Source: CAD feature listing. Evaluate the final solid. Frame: model axes, mm. Face numbers are marked on the shaded views. A direction names the side the tool comes from. Coordinates: 2 decimals unless noted, no trailing zeros. Write item = value, one per line. Start each with the question number.
1. Access query for the marked faces 1, 2 and 3. Directions: +Z, -Z, +X, -X, +Y, -Y. A direction counts if a zero-diameter tool reaches every point of the face in a straight line with its end or side. Return the directions, or none.
2. Line query: line 1 along Y through (x, z) = (-13.8, -17.5) (3 decimals); line 2 along X through (y, z) = (-13, -18.75); line 3 along Y through (x, z) = (15, -20.5) (3 decimals). Output: solid intervals per line, ascending.
3. Pin query (flat end, axial travel): pin 1 Ø1.3 at (y, z) = (4.5, -17.5) entering from -X; pin 2 Ø10 at (x, y) = (8.5, -12) entering from +Z; pin 3 Ø2.5 at (x, y) = (-7.78, -7.78) entering from +Z; pin 4 Ø1.1 at (x, z) = (13, -18) entering from +Y. Return the tip coordinate at first contact, or that it passes through.
4. Section query A-A (y = -3.5). Give the number of separate pieces and of enclosed holes in the cut face, then the cut area to 3 significant figures.
```python
from build123d import *

# Parameters (mm, degrees)
BOSS_EXTRUDE1_DEPTH              = 4.5
BOSS_EXTRUDE2_DEPTH              = 1.5
SKETCH3_W                        = 34.4
SKETCH3_H                        = 6
BOSS_EXTRUDE3_DEPTH              = 16.965402213
SKETCH4_W                        = 4.5
SKETCH4_H                        = 18
CUT_EXTRUDE1_DEPTH               = 24.8
SKETCH5_W                        = 4.8
SKETCH5_H                        = 6
BOSS_EXTRUDE4_DEPTH              = 4
SKETCH6_W                        = 4.8
SKETCH6_H                        = 6
BOSS_EXTRUDE5_DEPTH              = 4
SKETCH7_W                        = 4.5
SKETCH7_H                        = 12
CUT_EXTRUDE2_DEPTH               = 3.6
SKETCH8_W                        = 3.6
SKETCH8_H                        = 12
CUT_EXTRUDE3_DEPTH               = 4.5
F_2_05_2_05_DIAMETER_HOLE1_D     = 2.05
F_2_05_2_05_DIAMETER_HOLE1_DEPTH = 4.8
F_2_05_2_05_DIAMETER_HOLE2_D     = 2.05
F_2_5_2_5_DIAMETER_HOLE1_D       = 2.5
F_2_05_2_05_DIAMETER_HOLE3_D     = 2.05
F_2_05_2_05_DIAMETER_HOLE3_DEPTH = 6.000025
F_1_6_1_6_DIAMETER_HOLE1_D       = 1.6
F_1_6_1_6_DIAMETER_HOLE1_DEPTH   = 6.000025
F_8_0_8_DIAMETER_HOLE1_D         = 8
F_2_05_2_05_DIAMETER_HOLE4_D     = 2.05
F_2_05_2_05_DIAMETER_HOLE4_DEPTH = 9.5
CHAMFER1_SIZE                    = 0.3
CHAMFER2_SIZE2                   = 0.199958733
CHAMFER2_SIZE                    = 0.19995667
CHAMFER3_SIZE                    = 0.18964074
CHAMFER3_SIZE_2                  = 0.224716875
FILLET1_R                        = 1.5
FILLET2_R                        = 2


with BuildPart() as part:
    # Sketch1 → Boss-Extrude1 (new body)
    with BuildSketch(Plane.XY.offset(-15)):
        with BuildLine():
            Line((-17.2, 5.965402213), (17.2, 5.965402213))
            Line((17.2, 5.965402213), (15.505698966, 7.387089586))
            ThreePointArc((15.505698966, 7.387089586), (15.038810903, 7.100113286), (14.5, 7))
            Line((14.5, 7), (-14.5, 7))
            ThreePointArc((-14.5, 7), (-15.038810903, 7.100113286), (-15.505698966, 7.387089586))
            Line((-15.505698966, 7.387089586), (-17.2, 5.965402213))
        make_face()
    extrude(amount=-BOSS_EXTRUDE1_DEPTH)

    # Sketch2 → Boss-Extrude2 (add)
    with BuildSketch(Plane(origin=(0, 0, -19.5), x_dir=(-1, 0, 0), z_dir=(0, 0, -1))):
        Polygon((17.2, 5.965402213), (-17.2, 5.965402213), (-11.2, 11), (11.2, 11), align=None)
    extrude(amount=BOSS_EXTRUDE2_DEPTH)

    # Sketch3 → Boss-Extrude3 (add)
    with BuildSketch(Plane.XZ.offset(-5.965402213)):
        with Locations((0, -18)):
            Rectangle(SKETCH3_W, SKETCH3_H)
    extrude(amount=BOSS_EXTRUDE3_DEPTH)

    # Sketch4 → Cut-Extrude1 (cut)
    with BuildSketch(Plane(origin=(12.4, 0, 0), x_dir=(0, 0, -1), z_dir=(1, 0, 0))):
        with Locations((17.25, -2)):
            Rectangle(SKETCH4_W, SKETCH4_H)
    extrude(amount=-CUT_EXTRUDE1_DEPTH, mode=Mode.SUBTRACT)

    # Sketch5 → Boss-Extrude4 (add)
    with BuildSketch(Plane.XZ.offset(11)):
        with Locations((14.8, -18)):
            Rectangle(SKETCH5_W, SKETCH5_H)
    extrude(amount=BOSS_EXTRUDE4_DEPTH)

    # Sketch6 → Boss-Extrude5 (add)
    with BuildSketch(Plane.XZ.offset(11)):
        with Locations((-14.8, -18)):
            Rectangle(SKETCH6_W, SKETCH6_H)
    extrude(amount=BOSS_EXTRUDE5_DEPTH)

    # Sketch7 → Cut-Extrude2 (cut)
    with BuildSketch(Plane(origin=(-12.4, 0, 0), x_dir=(0, 0, -1), z_dir=(1, 0, 0))):
        with Locations((17.25, -4)):
            Rectangle(SKETCH7_W, SKETCH7_H)
    extrude(amount=-CUT_EXTRUDE2_DEPTH, mode=Mode.SUBTRACT)

    # Sketch8 → Cut-Extrude3 (cut)
    with BuildSketch(Plane.XY.offset(-15)):
        with Locations((14.2, -4)):
            Rectangle(SKETCH8_W, SKETCH8_H)
    extrude(amount=-CUT_EXTRUDE3_DEPTH, mode=Mode.SUBTRACT)

    # Ø2.05 (2.05) Diameter Hole1
    with Locations(Plane(origin=(-12.4, 0, 0), x_dir=(0, 0, -1), z_dir=(1, 0, 0))):
        with Locations((17.5, 4.5), (17.5, -12.5)):
            Hole(F_2_05_2_05_DIAMETER_HOLE1_D / 2, depth=F_2_05_2_05_DIAMETER_HOLE1_DEPTH)

    # Ø2.05 (2.05) Diameter Hole2 (through all)
    with Locations(Plane.ZY.offset(-12.4)):
        with Locations((-17.5, 4.5), (-17.5, -12.5)):
            Hole(F_2_05_2_05_DIAMETER_HOLE2_D / 2)

    # Ø2.5 (2.5) Diameter Hole1 (through all)
    with Locations(Plane.XY.offset(-19.5)):
        with Locations((3.5, 8), (-8, 3.5), (-3.5, -8), (8, -3.5)):
            Hole(F_2_5_2_5_DIAMETER_HOLE1_D / 2)

    # Ø2.05 (2.05) Diameter Hole3
    with Locations(Plane(origin=(0, 0, -21), x_dir=(-1, 0, 0), z_dir=(0, 0, -1))):
        with Locations((3.5, 8), (8, -3.5), (-3.5, -8), (-8, 3.5), (7.778174593, 7.778174593), (7.778174593, -7.778174593), (-7.778174593, -7.778174593), (-7.778174593, 7.778174593)):
            Hole(F_2_05_2_05_DIAMETER_HOLE3_D / 2, depth=F_2_05_2_05_DIAMETER_HOLE3_DEPTH)

    # Ø1.6 (1.6) Diameter Hole1
    with Locations(Plane(origin=(0, 0, -21), x_dir=(-1, 0, 0), z_dir=(0, 0, -1))):
        with Locations((0, 8), (-5.656854249, 5.656854249), (-8, 0), (-5.656854249, -5.656854249), (0, -8), (5.656854249, -5.656854249), (8, 0), (5.656854249, 5.656854249)):
            Hole(F_1_6_1_6_DIAMETER_HOLE1_D / 2, depth=F_1_6_1_6_DIAMETER_HOLE1_DEPTH)

    # Ø8.0 (8) Diameter Hole1 (through all)
    with Locations(Plane.XY.offset(-19.5)):
        with Locations((0, 0)):
            Hole(F_8_0_8_DIAMETER_HOLE1_D / 2)

    # Ø2.05 (2.05) Diameter Hole4
    with Locations(Plane.XY.offset(-15)):
        with Locations((15, 4.5), (-15, 4.5), (15, -12.5), (-15, -12.5)):
            Hole(F_2_05_2_05_DIAMETER_HOLE4_D / 2, depth=F_2_05_2_05_DIAMETER_HOLE4_DEPTH)

    # Chamfer1
    chamfer1_edges = [part.edges().sort_by_distance(p)[0] for p in [
        (12.4, -12.5, -15),
        (17.2, -12.5, -16.475),
        (17.2, 4.5, -16.475),
        (6.753174593, 7.778174593, -21),
        (6.753174593, -7.778174593, -21),
        (-8.803174593, -7.778174593, -21),
        (-8.803174593, 7.778174593, -21),
        (6.975, 3.5, -21),
        (2.475, -8, -21),
        (-9.025, -3.5, -21),
        (-4.525, 8, -21),
        (-6.456854249, 5.656854249, -21),
        (-8.8, 0, -21),
        (-6.456854249, -5.656854249, -21),
        (-0.8, -8, -21),
        (4.856854249, -5.656854249, -21),
        (7.2, 0, -21),
        (4.856854249, 5.656854249, -21),
        (-0.8, 8, -21),
        (-13.975, -12.5, -15),
        (16.025, -12.5, -15),
        (-13.975, 4.5, -15),
        (16.025, 4.5, -15),
        (17.2, -4.517298894, -15),
        (-17.2, -4.517298894, -15),
        (-17.2, -4.517298894, -21),
        (17.2, -4.517298894, -21),
        (-12.4, 4.5, -15),
        (12.4, 4.5, -15),
        (-12.4, -12.5, -15),
    ]]
    chamfer(chamfer1_edges, length=CHAMFER1_SIZE)

    # Chamfer2
    chamfer2_edges = [part.edges().sort_by_distance(p)[0] for p in [
        (4, 0, -21),
        (4, 0, -19.5),
    ]]
    chamfer(chamfer2_edges, length=CHAMFER2_SIZE, length2=CHAMFER2_SIZE2)

    # Chamfer3
    # the kernel refuses this chamfer: 0.224716875, 0.18964074 mm, written as the material it takes off along each edge
    with BuildSketch(Plane(origin=(15.505698966, 7.387089586, -14.344718434), x_dir=(0.7660444431190041, -0.6427876096865084, 0), z_dir=(0, 0, -1))) as chamfer3_piece_1:
        with BuildLine():
            Line((CHAMFER3_SIZE * 1.00000000217, 0), (-0.056208561, 0.248157995))
            ThreePointArc((-0.056208561, 0.248157995), (-0.023684334, 0.129009753), (0, 0))
            Line((0, 0), (CHAMFER3_SIZE * 1.00000000217, 0))
        make_face()
    extrude(amount=5.155281566, mode=Mode.SUBTRACT)
    with BuildSketch(Plane(origin=(-15.505698966, 7.387089586, -14.420065816), x_dir=(-0.7660444431188352, -0.6427876096867096, 0), z_dir=(0, 0, -1))) as chamfer3_piece_2:
        with BuildLine():
            Line((CHAMFER3_SIZE_2 * 0.999999998201, 0), (-0.041658025, -0.199529783))
            ThreePointArc((-0.041658025, -0.199529783), (-0.018131885, -0.103788276), (0, 0))
            Line((0, 0), (CHAMFER3_SIZE_2 * 0.999999998201, 0))
        make_face()
    extrude(amount=5.079934184, mode=Mode.SUBTRACT)

    # Fillet1
    fillet1_edges = [part.edges().sort_by_distance(p)[0] for p in [
        (16, 2, -17.25),
        (-16, -10, -17.25),
        (-16, 2, -17.25),
        (12.4, -11, -20.25),
        (16, -10, -17.25),
        (-12.4, -11, -20.25),
    ]]
    fillet(fillet1_edges, radius=FILLET1_R)

    # Fillet2
    fillet2_edges = [part.edges().sort_by_distance(p)[0] for p in [
        (11.2, 11, -20.25),
        (-11.2, 11, -20.25),
    ]]
    fillet(fillet2_edges, radius=FILLET2_R)


solid = part.part
```
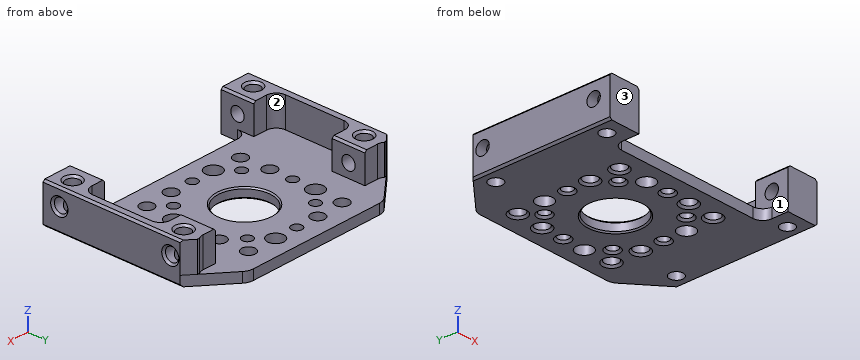
Results are:
q1.face_1 = +Z, -Y
q1.face_2 = +Z
q1.face_3 = +Z, -Z, +X, -X, -Y
q2.line_1 = -15 to -13.525, -11.475 to -10, 2 to 3.475, 5.525 to 7
q2.line_2 = -17.2 to -15.89, -14.11 to -12.4, 12.4 to 14.11, 15.89 to 17.2
q2.line_3 = -15 to -13.525, -11.475 to 3.475, 5.525 to 7.811
q3.pin_1 = through
q3.pin_2 = -15
q3.pin_3 = -19.5
q3.pin_4 = 7
q4.separate_pieces = 4
q4.enclosed_holes = 0
q4.area = 49.3 mm^2
